Design review of the part built by this model. Coordinates are the model's own, in mm. Face numbers are marked on the shaded views. Coordinates: 2 decimals unless noted, no trailing zeros. Loops run counter-clockwise (first coordinate to the right, second up) from the corner with the lowest first, then second, coordinate; pieces in that order, holes last.
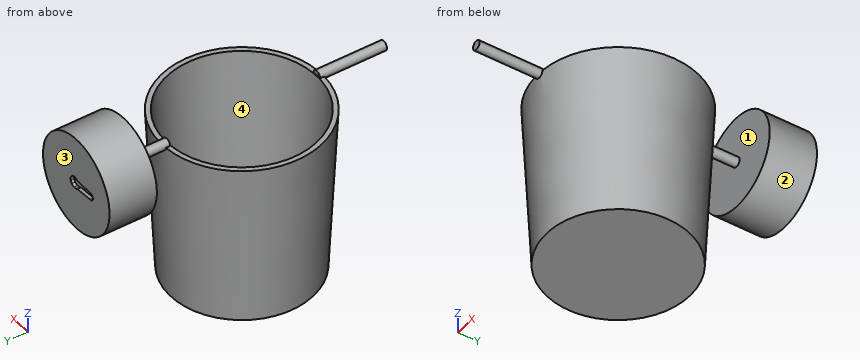
from build123d import *

# Parameters (mm, degrees)
EXTRUDE_DEPTH           = 4.5
EXTRUDE_PLACEMENT_ANGLE = 90
CYLINDER004_R           = 31.75
CYLINDER004_DEPTH       = 30
CYLINDER003_R           = 2
CYLINDER003_DEPTH       = 120
CYLINDER005_R           = 20
CYLINDER005_DEPTH       = 20


with BuildPart() as corona_servo:
    # path2399 → Extrude (new body)
    with BuildSketch(Plane(origin=(8.682374, -4.98127, 0), x_dir=(0, 1, 0), z_dir=(0, 0, 1))):
        with BuildLine():
            add(Edge.make_bspline(
                [(-1.415579, 5.024931), (-1.938341, -2.484397)],
                knots=[0, 0, 7.527502, 7.527502], degree=1))
            add(Edge.make_bspline(
                [(-1.938341, -2.484397), (-1.938341, -2.484397), (-2.134903, -2.858259), (-2.273136, -3.334737)],
                knots=[0, 0, 0, 0, 1, 1, 1, 1], degree=3))
            add(Edge.make_bspline(
                [(-2.273136, -3.334737), (-2.411369, -3.811216), (-2.443203, -4.128926), (-2.371685, -4.540758)],
                knots=[0, 0, 0, 0, 1, 1, 1, 1], degree=3))
            add(Edge.make_bspline(
                [(-2.371685, -4.540758), (-2.300167, -4.952591), (-2.218933, -5.672599), (-1.772797, -6.040394)],
                knots=[0, 0, 0, 0, 1, 1, 1, 1], degree=3))
            add(Edge.make_bspline(
                [(-1.772797, -6.040394), (-1.326661, -6.40819), (-0.861351, -6.572675), (-0.583202, -6.662312)],
                knots=[0, 0, 0, 0, 1, 1, 1, 1], degree=3))
            add(Edge.make_bspline(
                [(-0.583202, -6.662312), (-0.305053, -6.751952), (0.507781, -6.731952), (0.709843, -6.630052)],
                knots=[0, 0, 0, 0, 1, 1, 1, 1], degree=3))
            add(Edge.make_bspline(
                [(0.709843, -6.630052), (0.911905, -6.52815), (1.481843, -6.245909), (1.726833, -5.892641)],
                knots=[0, 0, 0, 0, 1, 1, 1, 1], degree=3))
            add(Edge.make_bspline(
                [(1.726833, -5.892641), (1.971823, -5.539373), (2.340182, -5.059724), (2.384256, -4.759981)],
                knots=[0, 0, 0, 0, 1, 1, 1, 1], degree=3))
            add(Edge.make_bspline(
                [(2.384256, -4.759981), (2.42833, -4.460237), (2.223091, -3.691858), (2.158411, -3.465999)],
                knots=[0, 0, 0, 0, 1, 1, 1, 1], degree=3))
            add(Edge.make_bspline(
                [(2.158411, -3.465999), (2.093732, -3.240141), (1.863634, -2.929328), (1.863634, -2.929328)],
                knots=[0, 0, 0, 0, 1, 1, 1, 1], degree=3))
            add(Edge.make_bspline(
                [(1.863634, -2.929328), (1.423808, 5.709855)],
                knots=[0, 0, 8.650371, 8.650371], degree=1))
            add(Edge.make_bspline(
                [(1.423808, 5.709855), (1.423808, 5.709855), (1.246198, 6.226563), (0.794563, 6.495307)],
                knots=[0, 0, 0, 0, 1, 1, 1, 1], degree=3))
            add(Edge.make_bspline(
                [(0.794563, 6.495307), (0.342929, 6.764051), (-0.057622, 6.753041), (-0.37358, 6.666974)],
                knots=[0, 0, 0, 0, 1, 1, 1, 1], degree=3))
            add(Edge.make_bspline(
                [(-0.37358, 6.666974), (-0.689538, 6.580907), (-1.208145, 6.230265), (-1.306201, 5.897514)],
                knots=[0, 0, 0, 0, 1, 1, 1, 1], degree=3))
            add(Edge.make_bspline(
                [(-1.306201, 5.897514), (-1.404257, 5.564763), (-1.415579, 5.024931), (-1.415579, 5.024931)],
                knots=[0, 0, 0, 0, 1, 1, 1, 1], degree=3))
        make_face()
    extrude(amount=EXTRUDE_DEPTH)


with BuildPart() as corona_servo_1:
    # Extrude placement: moved
    add(corona_servo.part.moved(Location((-12, 73, 75))).rotate(Axis((-12, 73, 75), (1, 0, 0)), EXTRUDE_PLACEMENT_ANGLE))


with BuildPart() as obj1:
    # Sketch → Revolution (revolve)
    with BuildSketch(Plane.XZ):
        Polygon((0, 1), (28, 1), (31.5, 70), (33.550725, 70), (30, 0), (0, 0), align=None)
    revolve(axis=Axis((0, 0, 0), (0, 0, 1)))


with BuildPart() as cylinder004:
    # Cylinder004 → Cylinder004 (new body)
    with BuildSketch(Plane.XY.offset(56)):
        Circle(CYLINDER004_R)
    extrude(amount=CYLINDER004_DEPTH)


with BuildPart() as cut001:
    # Cylinder003 → Cylinder003 (new body)
    with BuildSketch(Plane(origin=(0, 60, 70), x_dir=(1, 0, 0), z_dir=(0, -1, 0))):
        Circle(CYLINDER003_R)
    extrude(amount=CYLINDER003_DEPTH)

    # Cut001: cut Cylinder004
    add(cylinder004.part, mode=Mode.SUBTRACT)


with BuildPart() as cut:
    # Cylinder005 → Cylinder005 (new body)
    with BuildSketch(Plane(origin=(0, 70, 70), x_dir=(1, 0, 0), z_dir=(0, -1, 0))):
        Circle(CYLINDER005_R)
    extrude(amount=CYLINDER005_DEPTH)

    # Fusion: union Cut001
    add(cut001.part)

    # Fusion001: union obj1
    add(obj1.part)

    # Cut: cut corona_servo
    add(corona_servo_1.part, mode=Mode.SUBTRACT)


solid = cut.part
Q1. Take a section at C-C, the plane z = 39. Write out the cut boundary in (x, y).
Q2. Clearance check with flat-ended pins moving along their axes: pin 1 Ø8 at (y, z) = (-33, 30) entering from +X; pin 2 Ø5 at (x, z) = (25, 46.5) entering from -Y; pin 3 Ø2 at (x, z) = (7.5, 25.5) entering from -Y; pin 4 Ø5.5 at (x, z) = (-4, 69.5) entering from +Y. State where each tip first meets the part, or that it passes through.
Q3. Take a section at D-D, the plane y = -37. Write out the cut boundary in (x, z), then the cut area to 3 significant figures.
Q4. Take a section at B-B, the plane z = 80.5. Write out the cut boundary in (x, y).
Q5. Take a section at A-A, the plane y = 0. Write out the cut boundary in (x, z).
Q6. For line 1 (X direction, y = 10, z = 44.5); line 2 (X direction, y = 6.5, z = 14.5); line 3 (Y direction, x = 7, z = 64), list the stretches that pass through material, from the lowest coordinate up.
Q7. The part is to be moulded in two halves that separate along Y. For the marked faces 1, 2, 3 and 4, say which applies: pulls with the +Y half, pulls with the -Y half, needs draft (parallel to the pull), parting line crosses it, or undercut.
Entries:
1. outline: circle Ø63.96 at (0, 0); hole circle Ø59.86 at (0, 0)
2. pin 1: stops at x = 12.37
2. pin 2: stops at y = -23.26
2. pin 3: stops at y = -30.62
2. pin 4: stops at y = 70
3. outline: circle Ø4 at (0, 70)
3. area: 12.6 mm2
4. outline: (-17.02, 50) - (17.02, 50) - (17.02, 70) - (-17.02, 70) - close
5. outline: (-33.55, 70) - (-30, 0) - (30, 0) - (33.55, 70) - (31.5, 70) - (28, 1) - (-28, 1) - (-31.5, 70) - close
6. line 1: x = -30.67 to -28.5, 28.5 to 30.67
6. line 2: x = -30.04 to -27.94, 27.94 to 30.04
6. line 3: y = -32.5 to -30.4, 30.4 to 32.5, 50 to 70
7. face 1: undercut
7. face 2: needs draft
7. face 3: pulls with the +Y half
7. face 4: undercut
